```python
from build123d import *

# Parameters (mm, degrees)
SKETCH1_W                    = 93
SKETCH1_H                    = 20
BOSS_EXTRUDE1_DEPTH          = 6
CUT_EXTRUDE2_REACH           = 49.94
SKETCH3_W                    = 73
SKETCH3_H                    = 9
F_6_CLEARANCE_HOLE1_D        = 3.6576
TAP_DRILL_FOR_10_32_TAP1_D   = 4.0386
F_1_8_0_125_DIAMETER_HOLE1_D = 3.175
FILLET1_R                    = 1
CHAMFER2_SIZE                = 0.5


with BuildPart() as part:
    # Sketch1 → Boss-Extrude1 (new body)
    with BuildSketch(Plane.XY):
        Rectangle(SKETCH1_W, SKETCH1_H)
    extrude(amount=BOSS_EXTRUDE1_DEPTH)

    # Sketch3 → Cut-Extrude2 (cut, up to next)
    with BuildSketch(Plane.XY.offset(6), mode=Mode.PRIVATE) as cut_extrude2_sk1:
        with Locations((0, -5.5)):
            Rectangle(SKETCH3_W, SKETCH3_H)
    cut_extrude2_tool1 = extrude(cut_extrude2_sk1.sketch, amount=-CUT_EXTRUDE2_REACH, mode=Mode.PRIVATE) & part.part
    add(cut_extrude2_tool1.solids().sort_by_distance((0, -5.5, 6))[0], mode=Mode.SUBTRACT)

    # #6 Clearance Hole1 (through all)
    with Locations(Plane(origin=(0, -1, 0), x_dir=(-1, 0, 0), z_dir=(0, -1, 0))):
        with Locations((18, -3)):
            Hole(F_6_CLEARANCE_HOLE1_D / 2)

    # Tap Drill for #10-32 Tap1 (through all)
    with Locations(Plane.XY.offset(6)):
        with Locations((-42, -4), (42, -4)):
            Hole(TAP_DRILL_FOR_10_32_TAP1_D / 2)

    # 1/8 (0.125) Diameter Hole1 (through all)
    with Locations(Plane(origin=(0, -1, 0), x_dir=(-1, 0, 0), z_dir=(0, -1, 0))):
        with Locations((-18, -3)):
            Hole(F_1_8_0_125_DIAMETER_HOLE1_D / 2)

    # Fillet1
    fillet1_edges = [part.edges().sort_by_distance(p)[0] for p in [
        (-36.5, -10, 3),
        (-36.5, -1, 3),
        (36.5, -1, 3),
        (36.5, -10, 3),
        (46.5, -10, 3),
        (-46.5, -10, 3),
        (-46.5, 10, 3),
        (46.5, 10, 3),
    ]]
    fillet(fillet1_edges, radius=FILLET1_R)

    # Chamfer2
    chamfer2_edges = [part.edges().sort_by_distance(p)[0] for p in [
        (-19.8288, -1, 3),
        (-19.8288, 10, 3),
        (44.0193, -4, 6),
        (44.0193, -4, 0),
        (-39.9807, -4, 6),
        (-39.9807, -4, 0),
        (16.4125, -1, 3),
        (16.4125, 10, 3),
    ]]
    chamfer(chamfer2_edges, length=CHAMFER2_SIZE)


solid = part.part
```
The listing builds one solid part. Answer for the finished solid, in the listing's coordinates (mm). A direction names the side the tool comes from. Coordinates: 2 decimals unless noted, no trailing zeros. Write each loop counter-clockwise with the first axis right and the second up, starting at its lowest first coordinate (ties: lowest second). Pieces come first, ordered by that corner, then holes. Notation, with made-up numbers: (4.25, 79.5) - (23.25, 79.5) arc R26 cw to (23.25, 113.5) - close; hole circle Ø10 at (1.5, -7). An arc over 180 degrees is marked (long way). One line per item, written item: value.
1) A tool of negligible diameter and unlimited length cuts with its end or side. For faces 5 (the cylindrical face through (40.135, -4.773, 2.965)), 6 (the flat face through (0, -1, 3)), from which of +Z, -Z, +X, -X, +Y, -Y can it reach the whole face along a straight path? Write none if from no direction.
Geometry check:
face 5: +Z, -Z
face 6: +Z, -Z, -Y
2) This flat-tipped pin is pushed along its axis until it touches: pin 1 Ø6.5 at (x, y) = (42, -4) entering from +Z. Where does it stop, or does it pass through?
Geometry check:
pin 1: stops at z = 6
3) Find section C-C (x = 18). Give the vertices of the cut face in (y, z).
Geometry check:
outline: (-1, 0) - (10, 0) - (10, 0.91) - (9.5, 1.41) - (-0.5, 1.41) - (-1, 0.91) - close; (-1, 5.09) - (-0.5, 4.59) - (9.5, 4.59) - (10, 5.09) - (10, 6) - (-1, 6) - close
4) Find section D-D (y = 2.25). Give the vertices of the cut face in (x, z) (1 decimal), and give its area (3 significant figures).
Geometry check:
outline: (-46.5, 0) - (46.5, 0) - (46.5, 6) - (-46.5, 6) - close; hole circle Ø3.7 at (-18, 3); hole circle Ø3.2 at (18, 3)
area: 540 mm2
5) For a pull along X with two mould halves and no side action, classify faces 1 (the cylindrical face through (-43.865, -4.773, 2.965)), 2 (the flat face through (-1, 5, 6)), 3 (the flat face through (-46.5, 0, 3)), 4 (the flat face through (-36.5, -6, 3)) as pulls with the +X half, pulls with the -X half, needs draft (parallel to the pull), parting line crosses it, or undercut.
Geometry check:
face 1: undercut
face 2: needs draft
face 3: pulls with the -X half
face 4: undercut
6) Find section A-A (x = -42). Give the vertices of the cut face in (y, z).
Geometry check:
outline: (-10, 0) - (-6.52, 0) - (-6.02, 0.5) - (-6.02, 5.5) - (-6.52, 6) - (-10, 6) - close; (-1.98, 0.5) - (-1.48, 0) - (10, 0) - (10, 6) - (-1.48, 6) - (-1.98, 5.5) - close
7) Consider line 1 along X through (y, z) = (2, 3); line 2 along Y through (x, z) = (-42, 2.45); line 3 along Z through (x, y) = (-18, 6). Determine where each line is inside the solid, lowest interval first. Write a range as from..to.
Geometry check:
line 1: x = -46.5..-19.83, -16.17..16.41, 19.59..46.5
line 2: y = -10..-6.02, -1.98..10
line 3: z = 0..1.17, 4.83..6
8) Find section B-B (y = -4). Give the vertices of the cut face in (x, z).
Geometry check:
outline: (-46.5, 0) - (-44.52, 0) - (-44.02, 0.5) - (-44.02, 5.5) - (-44.52, 6) - (-46.5, 6) - close; (-39.98, 0.5) - (-39.48, 0) - (-36.5, 0) - (-36.5, 6) - (-39.48, 6) - (-39.98, 5.5) - close; (36.5, 0) - (39.48, 0) - (39.98, 0.5) - (39.98, 5.5) - (39.48, 6) - (36.5, 6) - close; (44.02, 0.5) - (44.52, 0) - (46.5, 0) - (46.5, 6) - (44.52, 6) - (44.02, 5.5) - close
